```python
from build123d import *

# Parameters (mm, degrees)
SKETCH7_R           = 381
BOSS_EXTRUDE3_DEPTH = 508
SKETCH8_R           = 444.5
BOSS_EXTRUDE4_DEPTH = 317.5


with BuildPart() as part:
    # Sketch7 → Boss-Extrude3 (new body)
    with BuildSketch(Plane.XY):
        Circle(SKETCH7_R)
    extrude(amount=BOSS_EXTRUDE3_DEPTH)

    # Sketch8 → Boss-Extrude4 (add)
    with BuildSketch(Plane.XY.offset(508)):
        with Locations(Location((0, 0, 0), (0, 0, 180))):
            Circle(SKETCH8_R)
    extrude(amount=BOSS_EXTRUDE4_DEPTH)

    # Sketch9 → Revolve1 (revolve)
    with BuildSketch(Plane.XY.offset(825.5)):
        with BuildLine():
            Line((0, 444.5), (0, -444.5))
            ThreePointArc((0, -444.5), (-444.5, 0), (0, 444.5))
        make_face()
    revolve(axis=Axis((0, 444.5, 825.5), (0, -1, 0)))


solid = part.part
```
Design review of the part built by this model. Coordinates are the model's own, in mm. A direction names the side the tool comes from. Give positions to 0.01 mm unless a question says otherwise; leave off trailing zeros. Write each loop counter-clockwise with the first axis right and the second up, starting at its lowest first coordinate (ties: lowest second). Pieces come first, ordered by that corner, then holes. Notation, with made-up numbers: (58.25, 39) -> (65.25, 39) arc R23 ccw to (65.25, 60) -> close; hole circle Ø7 at (80, -18). An arc over 180 degrees is marked (long way). Answer in a Markdown table with one row per item.
(1) Consider section D-D (z = 874.5). State the section outline as (x, y) points, then the cut area to 3 significant figures.
Results:
| item | result |
|---|---|
| outline | circle Ø883.58 at (0, 0) |
| area | 613,000 mm2 |
(2) For faces 1 (the cylindrical face through (-302.35, -231.83, 250.44)), 2 (the flat face through (-5, 5, 0)), list the 3-axis set-ups (+Z, -Z, +X, -X, +Y, -Y) from which the entire face can be reached by the end or side of a thin tool; tool diameter is ignored.
Results:
| item | result |
|---|---|
| face 1 | -Z |
| face 2 | -Z, +X, -X, +Y, -Y |
(3) Consider section A-A (y = 0). State the section outline as (x, z) points.
Results:
| item | result |
|---|---|
| outline | (-444.5, 508) -> (-381, 508) -> (-381, 0) -> (381, 0) -> (381, 508) -> (444.5, 508) -> (444.5, 825.5) arc R444.5 ccw to (-444.5, 825.5) -> close |
(4) To check wall thickness, follow probe 1 along Z at (x, y) = (-368, -185.5); probe 2 along Z at (x, y) = (-9, -389); probe 3 along Y at (x, z) = (-227, 974). State the ranges of each line that lie inside material, in increasing order.
Results:
| item | result |
|---|---|
| probe 1 | 508 to 992.07 |
| probe 2 | 508 to 1040.39 |
| probe 3 | -352.13 to 352.13 |
(5) Consider section C-C (z = 87.5). State the section outline as (x, y) points, then the cut area to 3 significant figures.
Results:
| item | result |
|---|---|
| outline | circle Ø762 at (0, 0) |
| area | 456,000 mm2 |
(6) Clearance check with flat-ended pins moving along their axes: pin 1 (5 mm diameter, centred on y = 56.5, z = 343, fed in from -X); pin 2 (8 mm diameter, centred on x = -309.5, z = 672, fed in from -Y); pin 3 (1.5 mm diameter, centred on x = 8.5, y = 310.5, fed in from +Z). State where each tip first meets the part, or that it passes through.
Results:
| item | result |
|---|---|
| pin 1 | x = -377.15 |
| pin 2 | y = -322.88 |
| pin 3 | z = 1144.19 |
